Work out the finished part from the listing and answer in its coordinate system (mm). Face numbers are marked on the shaded views. A direction names the side the tool comes from. Round coordinates to 2 decimals unless told otherwise and drop trailing zeros. Loops run counter-clockwise (first coordinate to the right, second up) from the corner with the lowest first, then second, coordinate; pieces in that order, holes last.
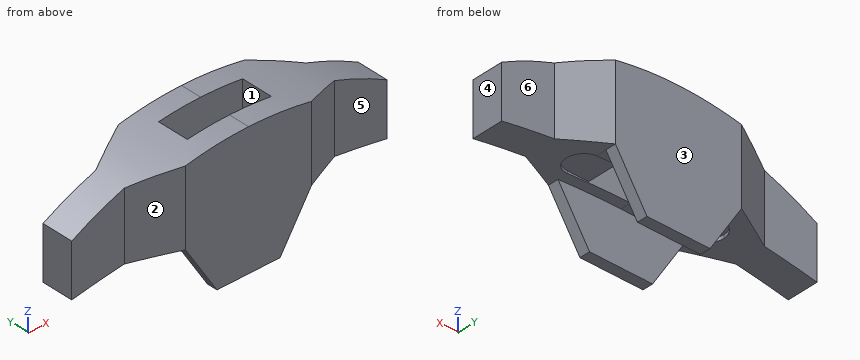
```python
from build123d import *

# Parameters (mm, degrees)
F2_DEPTH    = 3
F3_DEPTH    = 5
F4_START    = 5
F4_DEPTH    = 2
F5_T4_DEPTH = 55.7006365314
F5_S5_R     = 165
F5_T6_DEPTH = 30
F5_S7_R     = 61.9381694392
F5_T8_DEPTH = 30
F6_DEPTH    = 3
F7_R        = 2.99999


# Not quite as in the source:
# - a fillet or chamfer that OpenCascade refuses, or shapes differently, is made with other operations: its cross-section is extruded or revolved along the edge and cut away or added
# - a fillet or chamfer is up to 0.001 mm smaller than in the source, because OpenCascade refuses the exact size
# - a feature names something its author has since deleted; it is built from what else it names


with BuildPart() as f2:
    # F1 (on Front) → F2 (new body)
    with BuildSketch(Plane.XZ):
        with BuildLine():
            ThreePointArc((-30, -2.7501926041), (-21.0318278303, -1.3459068092), (-12, -0.4369421772))
            Line((-12, -0.4369421772), (-12, 13.8264323737))
            ThreePointArc((-12, 13.8264323737), (-21.2558932775, 11.2384911254), (-30, 7.2498073959))
            Line((-30, 7.2498073959), (-30, -2.7501926041))
        make_face()
        with BuildLine():
            ThreePointArc((-12, -0.4369421772), (-6.0039761506, -0.1092717271), (0, 0))
            Line((0, 0), (0, 15))
            ThreePointArc((0, 15), (-6.028624656, 14.7059099053), (-12, 13.8264323737))
            Line((-12, 13.8264323737), (-12, -0.4369421772))
        make_face()
    extrude(amount=F2_DEPTH)

    # F1 (on Front) → F3 (join)
    with BuildSketch(Plane.XZ):
        with BuildLine():
            ThreePointArc((-12, -0.4369421772), (-6.0039761506, -0.1092717271), (0, 0))
            Line((0, 0), (0, 15))
            ThreePointArc((0, 15), (-6.028624656, 14.7059099053), (-12, 13.8264323737))
            Line((-12, 13.8264323737), (-12, -0.4369421772))
        make_face()
    extrude(amount=F3_DEPTH)

    # F1 (on Front) → F4 (join)
    with BuildSketch(Plane.XZ.offset(F4_START)):
        with BuildLine():
            Line((0, -10), (0, 0))
            ThreePointArc((0, 0), (-6.0039761506, -0.1092717271), (-12, -0.4369421772))
            Line((-12, -0.4369421772), (-6, -10))
            Line((-6, -10), (0, -10))
        make_face()
        with BuildLine():
            ThreePointArc((-12, -0.4369421772), (-6.0039761506, -0.1092717271), (0, 0))
            Line((0, 0), (0, 15))
            ThreePointArc((0, 15), (-6.028624656, 14.7059099053), (-12, 13.8264323737))
            Line((-12, 13.8264323737), (-12, -0.4369421772))
        make_face()
    extrude(amount=F4_DEPTH)

    # F5: chamfer of 4 x 8 on 1 edges, made by hand


with BuildPart() as f5_tool2:
    # F5_s3 → F5_t4 (new body)
    with BuildSketch(Plane.XY.offset(-21.1555731675)):
        with BuildLine():
            Line((-11.7137832989, -7.1431083506), (-20.2862167011, -2.8568916494))
            Line((-20.2862167011, -2.8568916494), (-20.2862167011, -2.6968916494))
            ThreePointArc((-20.2862167011, -2.6968916494), (-16.1431083506, -2.84), (-12, -2.84))
            Line((-12, -2.84), (-11.84, -3))
            ThreePointArc((-11.84, -3), (-11.84, -5.0715541753), (-11.5537832989, -7.1431083506))
            Line((-11.5537832989, -7.1431083506), (-11.7137832989, -7.1431083506))
        make_face()
    extrude(amount=F5_T4_DEPTH)

    # F5_s5 → F5_t6 (cut, symmetric)
    with BuildSketch(Plane.XZ.offset(4.9)):
        with Locations((0, -165)):
            Circle(F5_S5_R)
    extrude(amount=F5_T6_DEPTH, both=True, mode=Mode.SUBTRACT)

    # F5_s7 → F5_t8 (intersect, symmetric)
    with BuildSketch(Plane.XZ.offset(4.9)):
        with Locations((0, -46.9381694392)):
            Circle(F5_S7_R)
    extrude(amount=F5_T8_DEPTH, both=True, mode=Mode.INTERSECT)

    split(bisect_by=Plane.XZ.offset(7), keep=Keep.BOTTOM)


with BuildPart() as f2_1:
    add(f2.part)

    # F5_t1: union F5_tool2
    add(f5_tool2.part)

    # F0 (on Front) → F6 (cut)
    with BuildSketch(Plane.XZ):
        Polygon((0, -20), (0, 0), (0, 110), (-6, 110), (-6, 100), (-8, 100), (-8, 0), (-15, 0), (-15, -20), align=None)
    extrude(amount=F6_DEPTH, mode=Mode.SUBTRACT)

    # F7 (radius 3 in the source; OpenCascade refuses exactly that, so slightly less here)
    f7_edges = [f2_1.edges().sort_by_distance(p)[0] for p in [
        (-15, -3, -0.341616),
    ]]
    fillet(f7_edges, radius=F7_R)

    # F8: F2 across plane


with BuildPart() as f2_2:
    add(f2_1.part)
    add(f2_1.part.mirror(Plane.XZ))

    # F9: F2 across plane


with BuildPart() as f2_3:
    add(f2_2.part)
    add(f2_2.part.mirror(Plane.YZ))


solid = f2_3.part
```
1. Determine the mould class of the marked faces 1, 2, 3 and 4 for opening direction Y: +Y half, -Y half, draft (parallel to the pull), parting line (faces both ways), or undercut.
Answer key:
face 1: undercut
face 2: -Y half
face 3: +Y half
face 4: draft
2. Find section D-D (z = -2). Write down the section's boundary in (x, y).
Answer key:
outline: (-30, -3) - (-25.61, -3) - (-25.61, 3) - (-30, 3) - close; (-11.02, -7) - (11.02, -7) - (11.02, -5) - (-11.02, -5) - close; (-11.02, 5) - (11.02, 5) - (11.02, 7) - (-11.02, 7) - close; (25.61, -3) - (30, -3) - (30, 3) - (25.61, 3) - close
3. Consider probe 1 along Y at (x, z) = (-4, 7); probe 2 along X at (y, z) = (0.25, 6.5); probe 3 along Y at (x, z) = (4, -0.75). Determine where each line is inside the solid, lowest interval first.
Answer key:
probe 1: y = -7 to -3, 3 to 7
probe 2: x = -30 to -8, 8 to 30
probe 3: y = -7 to -5, 5 to 7
4. Find section B-B (z = -6). Write down the section's boundary in (x, y), then the cut area to 3 significant figures.
Answer key:
outline: (-8.51, -7) - (8.51, -7) - (8.51, -5) - (-8.51, -5) - close; (-8.51, 5) - (8.51, 5) - (8.51, 7) - (-8.51, 7) - close
area: 68.1 mm2
5. Find section A-A (z = 2.25). Write down the section's boundary in (x, y), then the cut area to 3 significant figures.
Answer key:
outline: (-30, -3) - (-20, -3) - (-12, -7) - (12, -7) - (20, -3) - (30, -3) - (30, 3) - (20, 3) - (12, 7) - (-12, 7) - (-20, 3) - (-30, 3) - close; hole (-8, -3) - (8, -3) - (8, 3) - (-8, 3) - close
area: 520 mm2
6. Which of the six approach directions +Z, -Z, +X, -X, +Y, -Y give full straight-line access (tool end or side, diameter ignored) to the marked faces 5 and 6?
Answer key:
face 5: +Z, -Z, +X, -Y
face 6: +Z, -Z, +X, +Y
7. Find section C-C (x = -5). Write down the section's boundary in (y, z), then the cut area to 3 significant figures.
Answer key:
outline: (-7, -10) - (-5, -10) - (-5, -0.08) - (-3, -0.08) - (-3, 14.8) - (-7, 14.8) - close; (3, -0.08) - (5, -0.08) - (5, -10) - (7, -10) - (7, 14.8) - (3, 14.8) - close
area: 159 mm2
8. Given pin 1 (1.5 mm diameter, centred on y = -4.5, z = -4, fed in from +X); pin 2 (3 mm diameter, centred on x = -19.5, y = -4.5, fed in from -Z); pin 3 (5 mm diameter, centred on x = 20.5, y = 1.5, fed in from +Z), each flat-ended and moving along its own axis, determine where each tip first touches the part or whether it passes through.
Answer key:
pin 1: stops at x = 10.12
pin 2: stops at z = -1.2
pin 3: stops at z = 12.33
